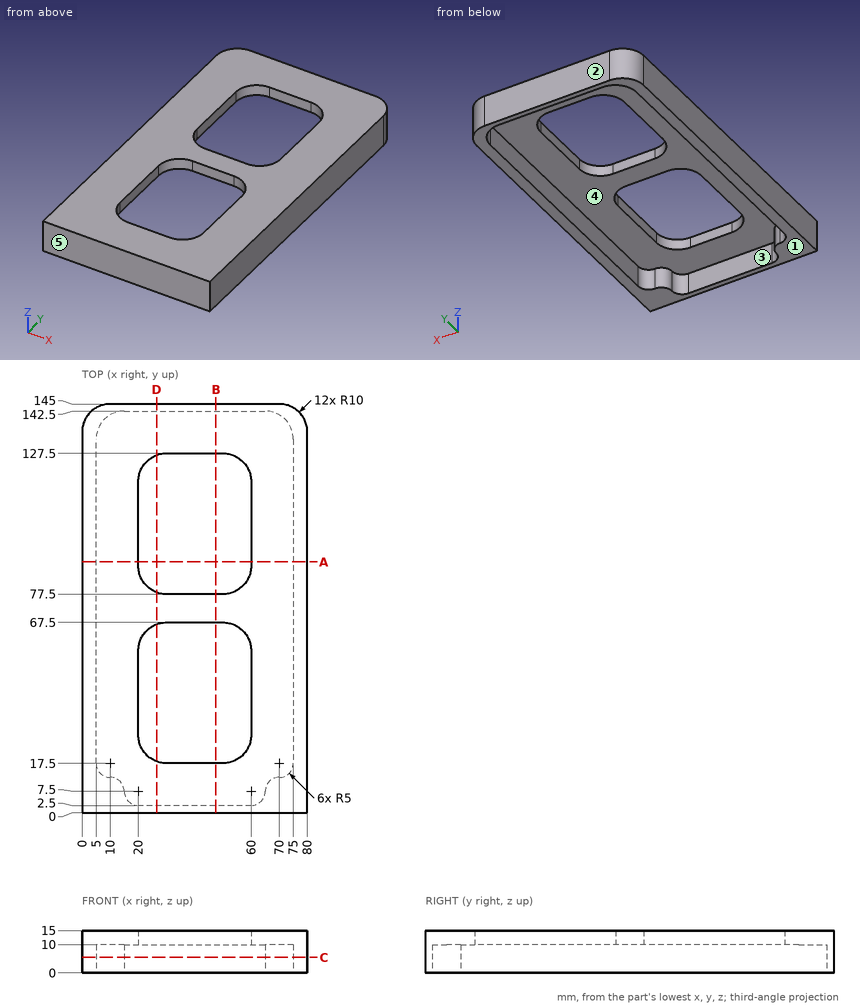
Print and shaded views of the part. All mm, measured from the part's lowest x, y and z. A direction names the side the tool comes from. Coordinates: 2 decimals unless noted, no trailing zeros. Order: outer loops, then holes, each group sorted by start corner. A loop starts at its lowest first (then second) coordinate and runs counter-clockwise, first axis right, second up. Notation, with made-up numbers: (56.5, -35.5) -> (97.5, -35.5) arc R28 cw to (97.5, -6.5) -> close; hole circle Ø3 at (51, 34.25). An arc over 180 degrees is marked (long way). Answer as a JSON object with one key per item and string values. Group by question number.
1) Pull direction Y, two halves, no side cores. Call the marked faces 1, 2 and 3: +Y half, -Y half, draft (parallel to the pull), parting line (faces both ways), or undercut.
2) Drill centre lines: L1, parallel to Y at x = 36, z = 13.75; L2, parallel to Y at x = 22.5, z = 3.25; L3, parallel to X at y = 97.5, z = 3.25. Where is each one in solid material? Low to high.
3) Which spindle directions (+Z, -Z, +X, -X, +Y, -Y) get a long thin tool onto all of the face, cutting with end or side? Do the marked faces 4 and 5. Say none if no direction does.
4) Cut at A-A, the plane y = 89. Write the cut outline in (x, z), then the cut area to 3 significant figures.
5) Cut at C-C, the plane z = 5.5. Write the cut outline in (x, y), then the cut area to 3 significant figures.
6) Cut at D-D, the plane x = 26.5. Write the cut outline in (y, z), then the cut area to 3 significant figures.
7) Cut at B-B, the plane x = 47.5. Write the cut outline in (y, z).
8) Flat gauge pins, fed straight in: pin 1 (5.5 mm diameter, centred on x = 41.5, z = 12.5, fed in from -Y); pin 2 (5 mm diameter, centred on x = 64.5, y = 98, fed in from -Z). Where does each tip first touch, or does it go through?
Check values:
{
 "1": {"face 1": "draft", "face 2": "+Y half", "face 3": "undercut"},
 "2": {"L1": "y = 0 to 17.5, 67.5 to 77.5, 127.5 to 145", "L2": "y = 0 to 2.5, 142.5 to 145", "L3": "x = 0 to 5, 75 to 80"},
 "3": {"face 4": "-Z", "face 5": "+Z, -Z, +X, -X, -Y"},
 "4": {"outline": "(0, 0) -> (5, 0) -> (5, 10) -> (20, 10) -> (20, 15) -> (0, 15) -> close; (60, 10) -> (75, 10) -> (75, 0) -> (80, 0) -> (80, 15) -> (60, 15) -> close", "area": "300 mm²"},
 "5": {"outline": "(0, 0) -> (80, 0) -> (80, 135) arc R10 ccw to (70, 145) -> (10, 145) arc R10 ccw to (0, 135) -> close; hole (5, 17.5) arc R5 ccw to (10, 12.5) arc R5 cw to (15, 7.5) arc R5 ccw to (20, 2.5) -> (60, 2.5) arc R5 ccw to (65, 7.5) arc R5 cw to (70, 12.5) arc R5 ccw to (75, 17.5) -> (75, 132.5) arc R10 ccw to (65, 142.5) -> (15, 142.5) arc R10 ccw to (5, 132.5) -> close", "area": "2,010 mm²"},
 "6": {"outline": "(0, 0) -> (2.5, 0) -> (2.5, 10) -> (18.13, 10) -> (18.13, 15) -> (0, 15) -> close; (66.87, 10) -> (78.13, 10) -> (78.13, 15) -> (66.87, 15) -> close; (126.87, 10) -> (142.5, 10) -> (142.5, 0) -> (145, 0) -> (145, 15) -> (126.87, 15) -> close", "area": "288 mm²"},
 "7": {"outline": "(0, 0) -> (2.5, 0) -> (2.5, 10) -> (17.5, 10) -> (17.5, 15) -> (0, 15) -> close; (67.5, 10) -> (77.5, 10) -> (77.5, 15) -> (67.5, 15) -> close; (127.5, 10) -> (142.5, 10) -> (142.5, 0) -> (145, 0) -> (145, 15) -> (127.5, 15) -> close"},
 "8": {"pin 1": "stops at y = 0", "pin 2": "stops at z = 10"}
}
